Part model, mm, in its own coordinate system. Face numbers are marked on the shaded views. A direction names the side the tool comes from. Round coordinates to 2 decimals unless told otherwise and drop trailing zeros. Write each loop counter-clockwise with the first axis right and the second up, starting at its lowest first coordinate (ties: lowest second). Pieces come first, ordered by that corner, then holes. Notation, with made-up numbers: M 13.5,54.5 L 52.5,54.5 A20 cw 52.5,81.5 Z; hole C 84.25,43 d10. An arc over 180 degrees is marked long. Answer as a JSON object with one key per item and string values. Group by question number.
1. Drill centre lines: line 1 (Y direction, x = 12.7, z = 1.9) (1 decimal); line 2 (Y direction, x = 19.5, z = 3.75) (3 decimals). Where is each one in solid material? Low to high. Write a range as from..to.
2. Band-saw the part on B-B, the plane z = 16.5. Write the cut outline in (x, y) (3 decimals).
3. Two-plate mould, pull along Y, no slides. Class the marked faces 3, 4, 5 and 6: +Y half, -Y half, draft (parallel to the pull), parting line (faces both ways), or undercut.
4. Band-saw the part on A-A, the plane x = 12.7. Write the cut outline in (y, z) (1 decimal), plus the area to 3 significant figures.
5. Drop a flat-ended pin along its axis: pin 1 (12.5 mm diameter, centred on x = 10, y = 14.5, fed in from +Z) (3 decimals). Give the stop position or say it passes through.
6. Which spindle directions (+Z, -Z, +X, -X, +Y, -Y) get a long thin tool onto all of the face, cutting with end or side? Do the marked faces 1 and 2. Say none if no direction does.
from build123d import *

# Parameters (mm, degrees)
F1_DEPTH = 22.225
F0_R     = 7.9375
F2_DEPTH = 3.175


with BuildPart() as f1:
    # F0 (on Top) → F1 (new body)
    with BuildSketch(Plane.XY):
        with BuildLine():
            Line((-3.175, 22.225), (-3.175, 12.7))
            Line((-3.175, 12.7), (-3.175, 3.175))
            ThreePointArc((-3.175, 3.175), (-1.315128, -1.315128), (3.175, -3.175))
            Line((3.175, -3.175), (12.7, -3.175))
            Line((12.7, -3.175), (22.225, -3.175))
            ThreePointArc((22.225, -3.175), (26.715128, -1.315128), (28.575, 3.175))
            Line((28.575, 3.175), (28.575, 12.7))
            Line((28.575, 12.7), (28.575, 22.225))
            ThreePointArc((28.575, 22.225), (26.715128, 26.715128), (22.225, 28.575))
            Line((22.225, 28.575), (12.7, 28.575))
            Line((12.7, 28.575), (3.175, 28.575))
            ThreePointArc((3.175, 28.575), (-1.315128, 26.715128), (-3.175, 22.225))
        make_face()
        with BuildLine():
            Line((0, 3.175), (0, 12.7))
            Line((0, 12.7), (0, 22.225))
            ThreePointArc((0, 22.225), (0.929936, 24.470064), (3.175, 25.4))
            Line((3.175, 25.4), (12.7, 25.4))
            Line((12.7, 25.4), (22.225, 25.4))
            ThreePointArc((22.225, 25.4), (24.470064, 24.470064), (25.4, 22.225))
            Line((25.4, 22.225), (25.4, 12.7))
            Line((25.4, 12.7), (25.4, 3.175))
            ThreePointArc((25.4, 3.175), (24.470064, 0.929936), (22.225, 0))
            Line((22.225, 0), (12.7, 0))
            Line((12.7, 0), (3.175, 0))
            ThreePointArc((3.175, 0), (0.929936, 0.929936), (0, 3.175))
        make_face(mode=Mode.SUBTRACT)
    extrude(amount=F1_DEPTH)

    # F0 (on Top) → F2 (join)
    with BuildSketch(Plane.XY):
        with BuildLine():
            Line((0, 22.225), (0, 12.7))
            Line((0, 12.7), (0, 3.175))
            ThreePointArc((0, 3.175), (0.929936, 0.929936), (3.175, 0))
            Line((3.175, 0), (12.7, 0))
            Line((12.7, 0), (22.225, 0))
            ThreePointArc((22.225, 0), (24.470064, 0.929936), (25.4, 3.175))
            Line((25.4, 3.175), (25.4, 12.7))
            Line((25.4, 12.7), (25.4, 22.225))
            ThreePointArc((25.4, 22.225), (24.470064, 24.470064), (22.225, 25.4))
            Line((22.225, 25.4), (12.7, 25.4))
            Line((12.7, 25.4), (3.175, 25.4))
            ThreePointArc((3.175, 25.4), (0.929936, 24.470064), (0, 22.225))
        make_face()
        with Locations((12.7, 12.7)):
            Circle(F0_R, mode=Mode.SUBTRACT)
    extrude(amount=F2_DEPTH)


solid = f1.part
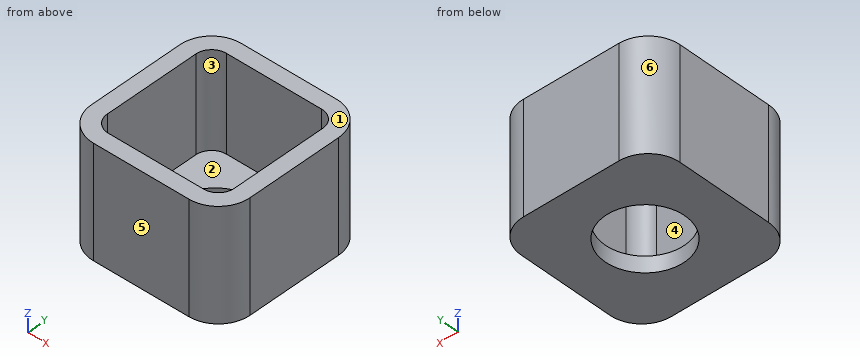
Worked answers:
{
 "1": {"line 1": "y = -3.2..4.8, 20.6..28.6", "line 2": "y = -3.175..0, 25.4..28.575"},
 "2": {"outline": "M -3.175,3.175 A6.35 ccw 3.175,-3.175 L 22.225,-3.175 A6.35 ccw 28.575,3.175 L 28.575,22.225 A6.35 ccw 22.225,28.575 L 3.175,28.575 A6.35 ccw -3.175,22.225 Z; hole M 0,3.175 A3.175 ccw 3.175,0 L 22.225,0 A3.175 ccw 25.4,3.175 L 25.4,22.225 A3.175 ccw 22.225,25.4 L 3.175,25.4 A3.175 ccw 0,22.225 Z"},
 "3": {"face 3": "undercut", "face 4": "undercut", "face 5": "-Y half", "face 6": "+Y half"},
 "4": {"outline": "M -3.2,0 L 4.8,0 L 4.8,3.2 L 0,3.2 L 0,22.2 L -3.2,22.2 Z; M 20.6,0 L 28.6,0 L 28.6,22.2 L 25.4,22.2 L 25.4,3.2 L 20.6,3.2 Z", "area": "171 mm^2"},
 "5": {"pin 1": "stops at z = 3.175"},
 "6": {"face 1": "+Z, +X, -X, +Y, -Y", "face 2": "+Z"}
}
